from build123d import *

# Parameters (mm, degrees)
BOSS_EXTRUDE1_DEPTH     = 25.4
BOSS_EXTRUDE1_2_DEPTH   = 25.4
CUT_EXTRUDE1_DEPTH      = 281.867791968
CUT_EXTRUDE1_DEPTH_BACK = 281.867791968
SKETCH2_OUTSIDE_W       = 232.096
SKETCH2_OUTSIDE_H       = 277.199
SKETCH2_OUTSIDE_W_2     = 46.910236734
SKETCH2_OUTSIDE_H_2     = 46.937556504


with BuildPart() as part:
    # Sketch1 → Boss-Extrude1 (new body)
    with BuildSketch(Plane(origin=(0, 0, 0), x_dir=(1, 0, 0), z_dir=(0, 1, 0))):
        with BuildLine():
            Line((0, 80.02759766), (0, 219.067642019))
            Line((0, 219.067642019), (103.040086398, 219.067642019))
            Line((103.040086398, 219.067642019), (103.040086398, 195.999460881))
            Line((103.040086398, 195.999460881), (23.011829096, 195.999460881))
            Line((23.011829096, 195.999460881), (23.011829096, 161.013213822))
            ThreePointArc((23.011829096, 161.013213822), (101.985495584, 126.901824422), (136.744902109, 48.211224327))
            ThreePointArc((136.744902109, 48.211224327), (146.280346481, 62.911008862), (150.026111113, 80.02759766))
            Line((150.026111113, 80.02759766), (150.026111113, 148.011746996))
            Line((150.026111113, 148.011746996), (172.974333949, 148.011746996))
            Line((172.974333949, 148.011746996), (172.974333949, 80.02759766))
            ThreePointArc((172.974333949, 80.02759766), (86.487166974, 0.037389651), (0, 80.02759766))
        make_face()
        with BuildLine():
            Line((23.011829096, 136.058182002), (23.011829096, 80.02759766))
            ThreePointArc((23.011829096, 80.02759766), (54.48283159, 31.69310754), (112.066438029, 28.410547154))
            ThreePointArc((112.066438029, 28.410547154), (90.841729512, 101.512108787), (23.011829096, 136.058182002))
        make_face(mode=Mode.SUBTRACT)
    extrude(amount=BOSS_EXTRUDE1_DEPTH)

    # Sketch2 outside → Cut-Extrude1 (cut, two sides: drawn at the far end of the back side and taken through both)
    with BuildSketch(Plane(origin=(0, 25.4, 0), x_dir=(1, 0, 0), z_dir=(0, 1, 0)).offset(-CUT_EXTRUDE1_DEPTH_BACK)):
        with Locations((86.964, 109.5525)):
            Rectangle(SKETCH2_OUTSIDE_W, SKETCH2_OUTSIDE_H)
        with Locations((150.472811492, 195.598863767)):
            Rectangle(SKETCH2_OUTSIDE_W_2, SKETCH2_OUTSIDE_H_2, mode=Mode.SUBTRACT)
    extrude(amount=CUT_EXTRUDE1_DEPTH + CUT_EXTRUDE1_DEPTH_BACK, mode=Mode.SUBTRACT)


with BuildPart() as body_2:
    # Sketch1 → Boss-Extrude1 2 (new body)
    with BuildSketch(Plane(origin=(0, 0, 0), x_dir=(1, 0, 0), z_dir=(0, 1, 0))):
        Polygon((173.927929859, 172.130085515), (150.026111113, 172.130085515), (150.026111113, 195.999460881), (127.017693125, 195.999460881), (127.017693125, 219.067642019), (173.927929859, 219.067642019), align=None)
    extrude(amount=BOSS_EXTRUDE1_2_DEPTH)


solid = body_2.part
Input: part model. Units: mm. Frame: model coordinates. A direction names the side the tool comes from. Give positions to 0.01 mm unless a question says otherwise; leave off trailing zeros. Loops run counter-clockwise (first coordinate to the right, second up) from the corner with the lowest first, then second, coordinate; pieces in that order, holes last. Notation, with made-up numbers: (72.5, 34.5) - (110.5, 34.5) arc R29 ccw to (110.5, 57.5) - close; hole circle Ø4 at (7, 14.25). An arc over 180 degrees is marked (long way). Use CSV: the item, a comma, the result in double quotes. Start each with the question number.
Item 1: Section B-B on z = -176. Return loops of the section in (x, y).
Item 2: Line query: line 1 (X direction, y = 16, z = -195); line 2 (Z direction, x = 140, y = 13.25). Output: solid intervals per line, ascending.
Item 3: Contact query for flat-ended pins moving along their axis: P1, Ø7, axis at x = 140, y = 16.5, coming from the +Z side; P2, Ø1, axis at y = 22.5, z = -180, coming from the -X side; P3, Ø3, axis at x = 141.5, z = -194, coming from the -Y side. Output: stop coordinate, or through.
Item 4: Reachability of faces 1 (the flat face through (162, 13, -172.13)), 2 (the flat face through (150.026, 13, -184)) from +Z, -Z, +X, -X, +Y, -Y: full face, straight path, thin tool, end or side. Return the list, or none.
Item 5: Section C-C on x = 142. Return loops of the section in (y, z), then the cut area to 3 significant figures.
Item 6: Section A-A on y = 17.25. Return loops of the section in (x, z).
Ans:
1,outline,"(150.03, 0) - (173.93, 0) - (173.93, 25.4) - (150.03, 25.4) - close"
2,line 1,"x = 150.03 to 173.93"
2,line 2,"z = -219.07 to -196"
3,P1,"stops at z = -196"
3,P2,"stops at x = 150.03"
3,P3,"passes through"
4,face 1,"+Z, +X, -X, +Y, -Y"
4,face 2,"+Z, -X, +Y, -Y"
5,outline,"(0, -219.07) - (25.4, -219.07) - (25.4, -196) - (0, -196) - close"
5,area,"586 mm2"
6,outline,"(127.02, -219.07) - (173.93, -219.07) - (173.93, -172.13) - (150.03, -172.13) - (150.03, -196) - (127.02, -196) - close"
